Part model, mm, in its own coordinate system. Give positions to 0.01 mm unless a question says otherwise; leave off trailing zeros. Loops run counter-clockwise (first coordinate to the right, second up) from the corner with the lowest first, then second, coordinate; pieces in that order, holes last. Notation, with made-up numbers: (36, -2.75) -> (69, -2.75) arc R13 ccw to (69, 7.25) -> close; hole circle Ø2 at (70.5, 66). An arc over 180 degrees is marked (long way). One line per question, with ' | ' between items.
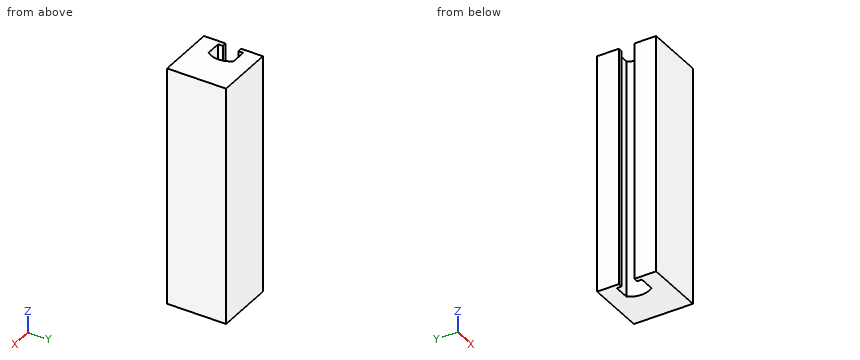
Solid Edge part; units mm, degrees
sketch "Sketch1" plane through (0, 0, 0) normal (0, 0, 1) x (1, 0, 0)
  line L0 (-10, -10) -> (10, -10)
  line L1 (10, -10) -> (10, 10)
  line L2 (10, 10) -> (-10, 10)
  line L3 (-10, 10) -> (-10, 2.65)
  line L4 (-8.5, 2.65) -> (-10, 2.65)
  line L5 (-8.5, 4.25) -> (-8.5, 2.65)
  line L6 (-3.3, 4.25) -> (-8.5, 4.25)
  arc A0 (-3.3, 4.25) -> (-3.3, -4.25) centre (-8.5833, 0) cw
  line L7 (-8.5, -4.25) -> (-3.3, -4.25)
  line L8 (-8.5, -2.65) -> (-8.5, -4.25)
  line L9 (-10, -2.65) -> (-8.5, -2.65)
  line L10 (-10, -2.65) -> (-10, -10)
extrude "Protrusion1" add sketch "Sketch1" along normal blind 81
1) Drill centre lines: line 1 (Y direction, x = -9, z = 31.5); line 2 (X direction, y = -3.25, z = 68.5); line 3 (Y direction, x = -8, z = 5). Where is each one in solid material? Low to high.
Found:
line 1: -10 to -2.65, 2.65 to 10 | line 2: -10 to -8.5, -2.63 to 10 | line 3: -10 to -4.25, 4.25 to 10
2) Saw through at A-A (x = -4). Give the cut face in (y, z).
Found:
outline: (-10, 0) -> (-4.25, 0) -> (-4.25, 81) -> (-10, 81) -> close; (4.25, 0) -> (10, 0) -> (10, 81) -> (4.25, 81) -> close
3) Saw through at B-B (z = 13). Give the cut face in (x, y), and give its area (3 significant figures).
Found:
outline: (-10, -10) -> (10, -10) -> (10, 10) -> (-10, 10) -> (-10, 2.65) -> (-8.5, 2.65) -> (-8.5, 4.25) -> (-3.3, 4.25) arc R6.78 cw to (-3.3, -4.25) -> (-8.5, -4.25) -> (-8.5, -2.65) -> (-10, -2.65) -> close | area: 339 mm2
